Answer from the drawing. Dimensions are ordinates in mm from the lowest x, y and z of the part. Coordinates: 2 decimals unless noted, no trailing zeros. Order: outer loops, then holes, each group sorted by start corner. A loop starts at its lowest first (then second) coordinate and runs counter-clockwise, first axis right, second up. Notation, with made-up numbers: M 9.25,-1.75 L 38.25,-1.75 A34 cw 38.25,28.25 Z; hole C 62.25,9.5 d7. An arc over 180 degrees is marked long. Write each question's results on one line, items separated by ' | '.
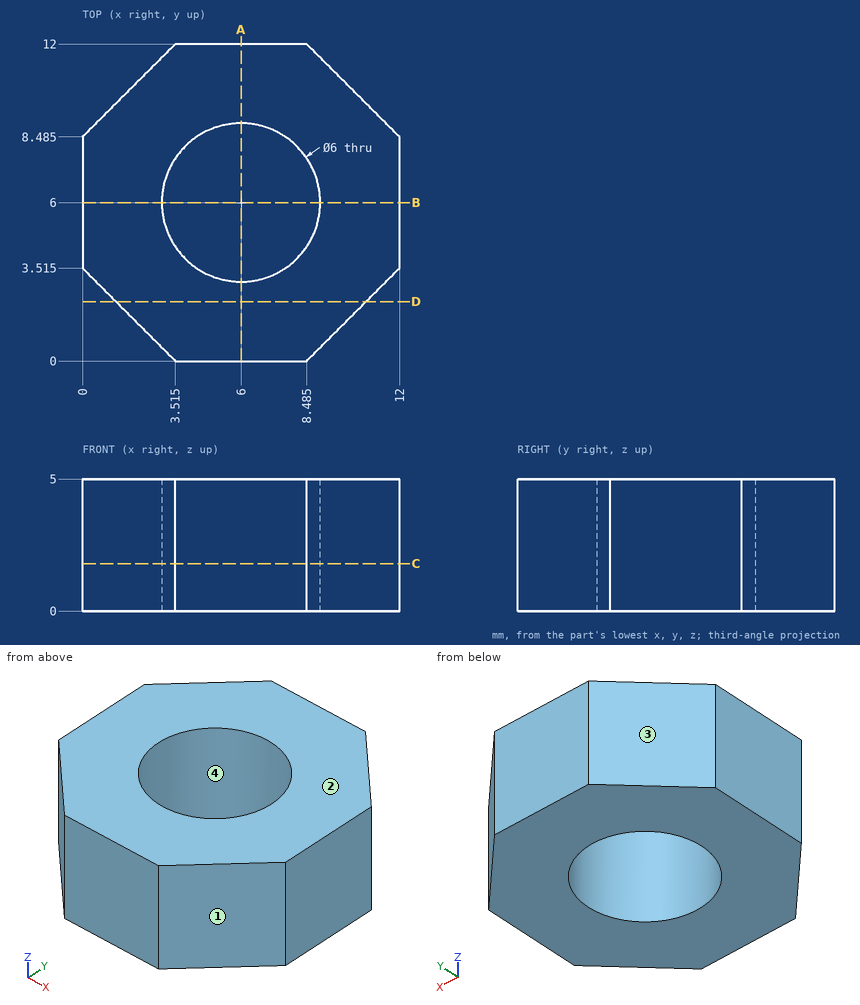
(1) Given pin 1 (3 mm diameter, centred on y = 7, z = 2.5, fed in from -X), flat-ended and moving along its own axis, determine where the tip first touches the part or whether it passes through.
Conclusion:
pin 1: x = 0
(2) Straight lines are drawn through the part: line 1 (Y direction, x = 6, z = 3.75); line 2 (X direction, y = 3.25, z = 0.3) (1 decimal); line 3 (Y direction, x = 4, z = 2.15) (1 decimal). For each, find the intervals that lie inside material, in ascending order.
Conclusion:
line 1: 0 to 3, 9 to 12 | line 2: 0.3 to 4.8, 7.2 to 11.7 | line 3: 0 to 3.8, 8.2 to 12
(3) The part is cut by section A-A, the plane x = 6. Write down the section's boundary in (y, z), then the cut area to 3 significant figures.
Conclusion:
outline: M 0,0 L 3,0 L 3,5 L 0,5 Z; M 9,0 L 12,0 L 12,5 L 9,5 Z | area: 30.0 mm²
(4) The part is cut by section D-D, the plane y = 2.25. Write down the section's boundary in (x, z) (1 decimal).
Conclusion:
outline: M 1.3,0 L 10.7,0 L 10.7,5 L 1.3,5 Z
(5) The part is cut by section C-C, the plane z = 1.8. Write down the section's boundary in (x, y) (1 decimal).
Conclusion:
outline: M 0,3.5 L 3.5,0 L 8.5,0 L 12,3.5 L 12,8.5 L 8.5,12 L 3.5,12 L 0,8.5 Z; hole C 6,6 d6
(6) The mould has two halves that part along Y. Classify the marked faces 1, 2, 3 and 4: pulls with the +Y half, pulls with the -Y half, needs draft (parallel to the pull), parting line crosses it, or undercut.
Conclusion:
face 1: pulls with the -Y half | face 2: needs draft | face 3: pulls with the +Y half | face 4: undercut
